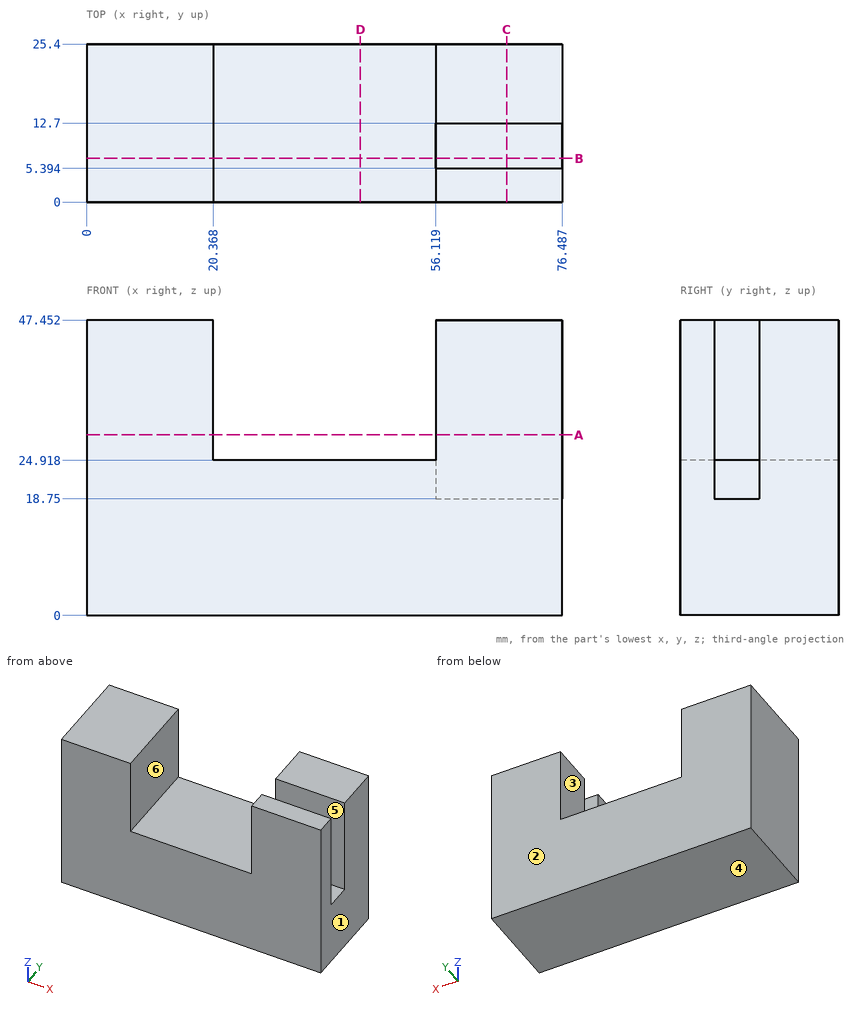
Drawing for the job (mm, zero at the part's lowest x, y, z). A direction names the side the tool comes from. Coordinates: 2 decimals unless noted, no trailing zeros. Loops run counter-clockwise (first coordinate to the right, second up) from the corner with the lowest first, then second, coordinate; pieces in that order, holes last. Notation, with made-up numbers: (-30.5, 56.25) - (-6.5, 56.25) arc R26 cw to (-6.5, 75.25) - close; hole circle Ø4 at (42, 89.25). An arc over 180 degrees is marked (long way). Use CSV: the item, a comma, the result in double quotes. Start each with the question number.
Q1. Cut at C-C, the plane x = 67.5. List the corners of the cut face in (y, z).
Q2. Probe probe 1 along X at (y, z) = (2.5, 37.5); probe 2 along Z at (x, y) = (43, 14.5); probe 3 along Y at (x, z) = (57.5, 37). List the from-to ranges inside material, lowest first. Write a range as from..to.
Q3. Drop a flat-ended pin along its axis: P1, Ø2, axis at x = 61.5, y = 9, coming from the +Z side. Give the stop position or say it passes through.
Q4. 3-axis set-ups, long thin cutter, end or side, ignore diameter. For the marked faces 4, 5 and 6: which of +Z, -Z, +X, -X, +Y, -Y reach the whole face in a straight line?
Q5. Two-plate mould, pull along X, no slides. Class the marked faces 1, 2 and 3: +X half, -X half, draft (parallel to the pull), parting line (faces both ways), or undercut.
Q6. Cut at D-D, the plane x = 44. List the corners of the cut face in (y, z).
Q7. Cut at B-B, the plane y = 7. List the corners of the cut face in (x, z), then the cut area to 3 significant figures.
Q8. Cut at A-A, the plane z = 29. List the corners of the cut face in (x, y).
Here are the results:
1,outline,"(0, 0) - (25.4, 0) - (25.4, 47.45) - (12.7, 47.45) - (12.7, 18.75) - (5.39, 18.75) - (5.39, 47.45) - (0, 47.45) - close"
2,probe 1,"0..20.37, 56.12..76.49"
2,probe 2,"0..24.92"
2,probe 3,"0..5.39, 12.7..25.4"
3,P1,"z = 18.75"
4,face 4,"-Z, +X, -X, +Y, -Y"
4,face 5,"+Z, +X"
4,face 6,"+Z, +Y, -Y"
5,face 1,"+X half"
5,face 2,"draft"
5,face 3,"undercut"
6,outline,"(0, 0) - (25.4, 0) - (25.4, 24.92) - (0, 24.92) - close"
7,outline,"(0, 0) - (76.49, 0) - (76.49, 18.75) - (56.12, 18.75) - (56.12, 24.92) - (20.37, 24.92) - (20.37, 47.45) - (0, 47.45) - close"
7,area,"2,240 mm2"
8,outline,"(0, 0) - (20.37, 0) - (20.37, 25.4) - (0, 25.4) - close; (56.12, 0) - (76.49, 0) - (76.49, 5.39) - (56.12, 5.39) - close; (56.12, 12.7) - (76.49, 12.7) - (76.49, 25.4) - (56.12, 25.4) - close"
